```python
from build123d import *

# Parameters (mm, degrees)
F1_DEPTH = 3.5
F2_R     = 2.875
F3_DEPTH = 3.5
F4_R     = 1


with BuildPart() as f1:
    # F0 (on Top) → F1 (new body)
    with BuildSketch(Plane.XY):
        with BuildLine():
            Line((-57, -50), (57, -50))
            ThreePointArc((57, -50), (59.12132, -49.12132), (60, -47))
            Line((60, -47), (60, 50))
            Line((60, 50), (-60, 50))
            Line((-60, 50), (-60, -47))
            ThreePointArc((-60, -47), (-59.12132, -49.12132), (-57, -50))
        make_face()
    extrude(amount=F1_DEPTH)

    # F2 (on face) → F3 (cut, through all)
    with BuildSketch(Plane.XY.offset(3.5)):
        with Locations((-53.75, 43.75)):
            Circle(F2_R)
        with Locations((53.75, 43.75)):
            Circle(F2_R)
        with Locations((-53.75, -43.75)):
            Circle(F2_R)
        with Locations((53.75, -43.75)):
            Circle(F2_R)
    extrude(amount=-F3_DEPTH, mode=Mode.SUBTRACT)

    # F4
    f4_edges = [f1.edges().sort_by_distance(p)[0] for p in [
        (0, -50, 3.5),
        (-59.12132, -49.12132, 3.5),
        (-60, 1.5, 3.5),
        (0, 50, 3.5),
        (60, 1.5, 3.5),
        (59.12132, -49.12132, 3.5),
    ]]
    fillet(f4_edges, radius=F4_R)


solid = f1.part
```
Design review of the part built by this model. Coordinates are the model's own, in mm. Give positions to 0.01 mm unless a question says otherwise; leave off trailing zeros. Order: outer loops, then holes, each group sorted by start corner. A loop starts at its lowest first (then second) coordinate and runs counter-clockwise, first axis right, second up. Notation, with made-up numbers: M -8,2 L 3,2 A23 ccw 3,22 Z; hole C 84.5,87.5 d10. An arc over 180 degrees is marked long. One line per question, with ' | ' between items. Start each with the question number.
Q1. For L1, parallel to Y at x = 53.75, z = 1.8 (3 decimals); L2, parallel to Y at x = -4, z = 2.55; L3, parallel to Y at x = 44, z = 3.05, list the stretches that pass through material, from the lowest coordinate up. Write a range as [from, to].
Q2. We need section B-B (x = 53.75). Write out the cut boundary in (y, z) (3 decimals).
Q3. We need section A-A (y = -43.75). Write out the cut boundary in (x, z) (3 decimals).
Returned:
1) L1: [-50, -46.625], [-40.875, 40.875], [46.625, 50] | L2: [-50, 50] | L3: [-49.84, 49.84]
2) outline: M -50,0 L -46.625,0 L -46.625,3.5 L -49,3.5 A1 ccw -50,2.5 Z; M -40.875,0 L 40.875,0 L 40.875,3.5 L -40.875,3.5 Z; M 46.625,0 L 50,0 L 50,2.5 A1 ccw 49,3.5 L 46.625,3.5 Z
3) outline: M -60,0 L -56.625,0 L -56.625,3.5 L -59,3.5 A1 ccw -60,2.5 Z; M -50.875,0 L 50.875,0 L 50.875,3.5 L -50.875,3.5 Z; M 56.625,0 L 60,0 L 60,2.5 A1 ccw 59,3.5 L 56.625,3.5 Z
